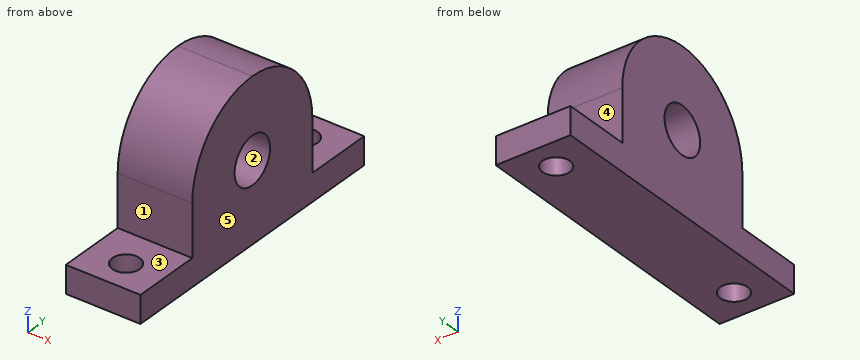
from build123d import *

# Parameters (mm, degrees)
F0_W      = 119.8626
F0_H      = 64.2874
F1_DEPTH  = 30.1625
F2_R      = 9.525
F3_DEPTH  = 30.1635
F7_DEPTH  = 30.1635
F8_DEPTH  = 30.1635
F9_R      = 5.55625
F10_DEPTH = 32.1447


with BuildPart() as f1:
    # F0 (on Right) → F1 (new body)
    with BuildSketch(Plane.YZ):
        Rectangle(F0_W, F0_H)
    extrude(amount=F1_DEPTH)

    # F2 (on face) → F3 (cut, through all)
    with BuildSketch(Plane.YZ.offset(30.1625)):
        Circle(F2_R)
    extrude(amount=-F3_DEPTH, mode=Mode.SUBTRACT)

    # F5 (on face) → F7 (cut, through all)
    with BuildSketch(Plane.YZ.offset(30.1625)):
        with BuildLine():
            ThreePointArc((-32.1437, 0), (-22.72902828, 22.7290282049), (-1.062e-07, 32.1437))
            Line((-1.062e-07, 32.1437), (-59.9313, 32.1437))
            Line((-59.9313, 32.1437), (-59.9313, -21.0312))
            Line((-59.9313, -21.0312), (-32.1437, -21.0312))
            Line((-32.1437, -21.0312), (-32.1437, 0))
        make_face()
    extrude(amount=-F7_DEPTH, mode=Mode.SUBTRACT)

    # F6 (on face) → F8 (cut, through all)
    with BuildSketch(Plane.YZ.offset(30.1625)):
        with BuildLine():
            Line((59.9313, 32.1437), (-1.062e-07, 32.1437))
            ThreePointArc((-1.062e-07, 32.1437), (22.7290282049, 22.72902828), (32.1437, 0))
            Line((32.1437, 0), (32.1437, -21.0312))
            Line((32.1437, -21.0312), (59.9313, -21.0312))
            Line((59.9313, -21.0312), (59.9313, 32.1437))
        make_face()
    extrude(amount=-F8_DEPTH, mode=Mode.SUBTRACT)

    # F9 (on Top) → F10 (cut, through all)
    with BuildSketch(Plane.XY):
        with Locations((15.0622, -47.625)):
            Circle(F9_R)
        with Locations((15.0622, 47.625)):
            Circle(F9_R)
    extrude(amount=-F10_DEPTH, mode=Mode.SUBTRACT)


solid = f1.part
Could you check a few things on this model? Use its own coordinates, in mm. Face numbers are marked on the shaded views. A direction names the side the tool comes from. Give positions to 0.01 mm unless a question says otherwise; leave off trailing zeros. Order: outer loops, then holes, each group sorted by start corner. A loop starts at its lowest first (then second) coordinate and runs counter-clockwise, first axis right, second up.
1. Will these pins go through, and if not, where does the flat tip stop? P1, Ø1.5, axis at x = 17, y = 44.5, coming from the +Z side; P2, Ø8.5, axis at x = 15.5, y = 51, coming from the +Z side; P3, Ø17, axis at x = 21, z = -12.5, coming from the +Y side; P4, Ø1.5, axis at x = 16, z = 18, coming from the +Y side.
2. For the marked faces 4 and 5, which set-ups out of +Z, -Z, +X, -X, +Y, -Y let a thin tool reach every point of the face, with its end or its side?
3. Suppose I cut it at B-B (x = 28.5). List the corners of the cut face in (y, z) for me (3 decimals).
4. We'd pull the mould along Y, two halves only. Please class the marked faces 1, 2 and 3: pulls with the +Y half, pulls with the -Y half, needs draft (parallel to the pull), parting line crosses it, or undercut.
5. Suppose I cut it at C-C (z = 21.5). List the corners of the cut face in (x, y) for me, plus the area to 3 significant figures.
6. Suppose I cut it at D-D (y = 29). List the corners of the cut face in (x, z) for me, plus the area to 3 significant figures.
7. Suppose I cut it at A-A (x = 14). List the corners of the cut face in (y, z) for me (3 decimals), plus the area to 3 significant figures.
8. I need wall thicknesses on L1, parallel to Z at x = 23, y = 0 (3 decimals); L2, parallel to Y at x = 16, z = -26; L3, parallel to Z at x = 18.5, y = -37.5. Which ranges of each line are inside material? Lowest first, please.
Solved:
1. P1: passes through
1. P2: stops at z = -21.03
1. P3: stops at y = 32.14
1. P4: stops at y = 27.12
2. face 4: +Z, +X, -X, +Y
2. face 5: +Z, -Z, +X, +Y, -Y
3. outline: (-59.931, -32.144) - (59.931, -32.144) - (59.931, -21.031) - (32.144, -21.031) - (32.144, 0) arc R32.144 ccw to (-32.144, 0) - (-32.144, -21.031) - (-59.931, -21.031) - close; hole circle Ø19.05 at (0, 0)
4. face 1: pulls with the -Y half
4. face 2: undercut
4. face 3: needs draft
5. outline: (0, -23.89) - (30.16, -23.89) - (30.16, 23.89) - (0, 23.89) - close
5. area: 1,440 mm2
6. outline: (0, -32.14) - (30.16, -32.14) - (30.16, 13.86) - (0, 13.86) - close
6. area: 1,390 mm2
7. outline: (-59.931, -32.144) - (-53.079, -32.144) - (-53.079, -21.031) - (-59.931, -21.031) - close; (-42.171, -32.144) - (42.171, -32.144) - (42.171, -21.031) - (32.144, -21.031) - (32.144, 0) arc R32.144 ccw to (-32.144, 0) - (-32.144, -21.031) - (-42.171, -21.031) - close; (53.079, -32.144) - (59.931, -32.144) - (59.931, -21.031) - (53.079, -21.031) - close; hole circle Ø19.05 at (0, 0)
7. area: 3,780 mm2
8. L1: z = -32.144 to -9.525, 9.525 to 32.144
8. L2: y = -59.93 to -53.1, -42.15 to 42.15, 53.1 to 59.93
8. L3: z = -32.14 to -21.03
